Work out the finished part from the listing and answer in its coordinate system (mm). Round coordinates to 2 decimals unless told otherwise and drop trailing zeros. Order: outer loops, then holes, each group sorted by start corner. A loop starts at its lowest first (then second) coordinate and runs counter-clockwise, first axis right, second up. Notation, with made-up numbers: (17, 87.5) -> (73, 87.5) arc R13 cw to (73, 110.5) -> close; hole circle Ø8 at (-27.5, -13). An arc over 180 degrees is marked (long way). Use one line per item in the form item = value.
Solid Edge part; units mm, degrees
sketch "Sketch1" plane through (0, 0, 0) normal (0, -1, 0) x (1, 0, 0)
  circle A0 centre (0, 0) radius 4.5
  circle A1 centre (-5.5, 24) radius 1.6
  circle A2 centre (5.5, 24) radius 1.6
  circle A3 centre (-5.5, -24) radius 1.6
  circle A4 centre (5.5, -24) radius 1.6
  line L0 (-9, -27.5) -> (9, -27.5)
  line L1 (9, -27.5) -> (9, 27.5)
  line L2 (9, 27.5) -> (-9, 27.5)
  line L3 (-9, 27.5) -> (-9, -27.5)
  dimension "D1" = 9
  dimension "D2" = 9
extrude "Protrusion1" add sketch "Sketch1" along normal blind 6
sketch "Sketch2" plane through (0, -6, 0) normal (0, -1, 0) x (1, 0, 0)
  circle A0 centre (0, 0) radius 6.5
extrude "ExtrudedCutout_1" cut sketch "Sketch2" against normal blind 2.5
hole "Hole_5" at (-5, 0, -7.5) direction (0, -1, 0) diameter 2.459 end up to next
hole "Hole1" at (-5, 0, 7.5) direction (0, -1, 0) diameter 2.459 end up to next
hole "Hole2" at (5, 0, 7.5) direction (0, -1, 0) diameter 2.459 end up to next
hole "Hole3" at (5, 0, -7.5) direction (0, -1, 0) diameter 2.459 end up to next
sketch "Sketch3" plane through (0, 0, 0) normal (0, 1, 0) x (-1, 0, 0)
  circle A0 centre (-5.5, -24) radius 2.9
  circle A1 centre (5.5, -24) radius 2.9
  circle A2 centre (5.5, 24) radius 2.9
  circle A3 centre (-5.5, 24) radius 2.9
extrude "ExtrudedCutout_2" cut sketch "Sketch3" against normal blind 3
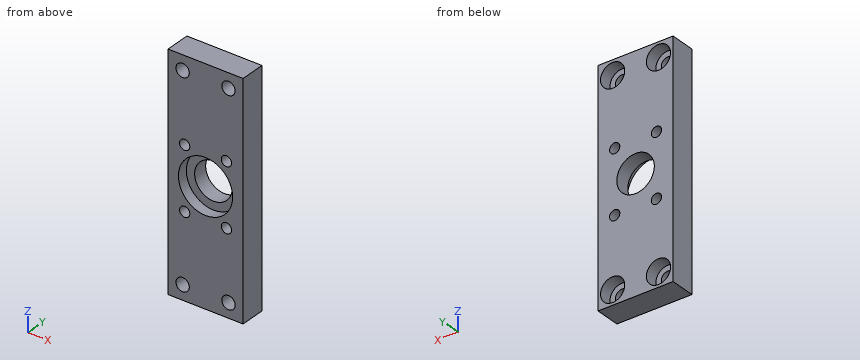
Item 1: Consider line 1 along X through (y, z) = (-5.05, -24); line 2 along X through (y, z) = (-1.65, 0); line 3 along Z through (x, y) = (5.5, -4.35). Determine where each line is inside the solid, lowest interval first.
Findings:
line_1 = -9 to -7.1, -3.9 to 3.9, 7.1 to 9
line_2 = -9 to -4.5, 4.5 to 9
line_3 = -27.5 to -25.6, -22.4 to -8.62, -6.38 to -3.46, 3.46 to 6.38, 8.62 to 22.4, 25.6 to 27.5
Item 2: The part is cut by section A-A, the plane z = 7.5. Give the vertices of the cut face in (x, y).
Findings:
outline = (-9, -6) -> (-6.23, -6) -> (-6.23, 0) -> (-9, 0) -> close; (-3.77, -6) -> (3.77, -6) -> (3.77, 0) -> (-3.77, 0) -> close; (6.23, -6) -> (9, -6) -> (9, 0) -> (6.23, 0) -> close
Item 3: A flat-ended cylindrical pin translates along its axis: P1, Ø3, axis at x = -5, z = -25, coming from the +Y side. Find the tip coordinate at first contact, or state that the pin passes through.
Findings:
P1 = -3
Item 4: The part is cut by section C-C, the plane y = -5.5. Give the number of separate pieces and of enclosed holes in the cut face, and give its area (3 significant figures).
Findings:
separate_pieces = 1
enclosed_holes = 9
area = 806 mm^2
Item 5: The part is cut by section B-B, the plane z = 0. Give the vertices of the cut face in (x, y).
Findings:
outline = (-9, -6) -> (-6.5, -6) -> (-6.5, -3.5) -> (-4.5, -3.5) -> (-4.5, 0) -> (-9, 0) -> close; (4.5, -3.5) -> (6.5, -3.5) -> (6.5, -6) -> (9, -6) -> (9, 0) -> (4.5, 0) -> close
